from build123d import *

# Parameters (mm, degrees)
F0_R     = 3.175
F1_DEPTH = 12.7
F2_DEPTH = 19.05
F3_R     = 5.08


with BuildPart() as f1:
    # F0 (on Top) → F1 (new body)
    with BuildSketch(Plane.XY):
        with BuildLine():
            Line((21.2967025781, 50.8), (-38.3932974219, 50.8))
            Line((-38.3932974219, 50.8), (-38.3932974219, -6.35))
            Line((-38.3932974219, -6.35), (21.2967025781, -6.35))
            Line((21.2967025781, -6.35), (21.2967025781, -3.175))
            ThreePointArc((21.2967025781, -3.175), (19.0516385478, -2.2450640303), (18.1217025781, 0))
            ThreePointArc((18.1217025781, 0), (21.2967025781, 3.175), (24.4717025781, 0))
            Line((24.4717025781, 0), (31.4567025781, 0))
            Line((31.4567025781, 0), (31.4567025781, 44.45))
            Line((31.4567025781, 44.45), (24.4717025781, 44.45))
            ThreePointArc((24.4717025781, 44.45), (21.2967025781, 41.275), (18.1217025781, 44.45))
            ThreePointArc((18.1217025781, 44.45), (19.0516385478, 46.6950640303), (21.2967025781, 47.625))
            Line((21.2967025781, 47.625), (21.2967025781, 50.8))
        make_face()
        Circle(F0_R, mode=Mode.SUBTRACT)
        with BuildLine():
            ThreePointArc((7.473351289, 0), (10.648351289, 3.175), (13.823351289, 0))
            ThreePointArc((13.823351289, 0), (10.648351289, -3.175), (7.473351289, 0))
        make_face(mode=Mode.SUBTRACT)
        with Locations((0, 44.45)):
            Circle(F0_R, mode=Mode.SUBTRACT)
        with BuildLine():
            ThreePointArc((7.473351289, 44.45), (10.648351289, 47.625), (13.823351289, 44.45))
            ThreePointArc((13.823351289, 44.45), (10.648351289, 41.275), (7.473351289, 44.45))
        make_face(mode=Mode.SUBTRACT)
        with BuildLine():
            Line((31.4567025781, 50.8), (21.2967025781, 50.8))
            Line((21.2967025781, 50.8), (21.2967025781, 47.625))
            ThreePointArc((21.2967025781, 47.625), (23.5417666083, 46.6950640303), (24.4717025781, 44.45))
            Line((24.4717025781, 44.45), (31.4567025781, 44.45))
            Line((31.4567025781, 44.45), (31.4567025781, 50.8))
        make_face()
        with BuildLine():
            Line((21.2967025781, -3.175), (21.2967025781, -6.35))
            Line((21.2967025781, -6.35), (31.4567025781, -6.35))
            Line((31.4567025781, -6.35), (31.4567025781, 0))
            Line((31.4567025781, 0), (24.4717025781, 0))
            ThreePointArc((24.4717025781, 0), (23.5417666083, -2.2450640303), (21.2967025781, -3.175))
        make_face()
    extrude(amount=-F1_DEPTH)

    # F0 (on Top) → F2 (join)
    with BuildSketch(Plane.XY):
        Circle(F0_R)
        with BuildLine():
            ThreePointArc((7.473351289, 0), (10.648351289, -3.175), (13.823351289, 0))
            Line((13.823351289, 0), (7.473351289, 0))
        make_face()
        with BuildLine():
            Line((7.473351289, 0), (13.823351289, 0))
            ThreePointArc((13.823351289, 0), (10.648351289, 3.175), (7.473351289, 0))
        make_face()
        with BuildLine():
            ThreePointArc((24.4717025781, 0), (21.2967025781, 3.175), (18.1217025781, 0))
            Line((18.1217025781, 0), (21.2967025781, 0))
            Line((21.2967025781, 0), (24.4717025781, 0))
        make_face()
        with BuildLine():
            ThreePointArc((18.1217025781, 0), (19.0516385478, -2.2450640303), (21.2967025781, -3.175))
            Line((21.2967025781, -3.175), (21.2967025781, 0))
            Line((21.2967025781, 0), (18.1217025781, 0))
        make_face()
        with BuildLine():
            Line((21.2967025781, 0), (21.2967025781, -3.175))
            ThreePointArc((21.2967025781, -3.175), (23.5417666083, -2.2450640303), (24.4717025781, 0))
            Line((24.4717025781, 0), (21.2967025781, 0))
        make_face()
        with Locations((0, 44.45)):
            Circle(F0_R)
        with BuildLine():
            ThreePointArc((7.473351289, 44.45), (10.648351289, 41.275), (13.823351289, 44.45))
            Line((13.823351289, 44.45), (7.473351289, 44.45))
        make_face()
        with BuildLine():
            Line((7.473351289, 44.45), (13.823351289, 44.45))
            ThreePointArc((13.823351289, 44.45), (10.648351289, 47.625), (7.473351289, 44.45))
        make_face()
        with BuildLine():
            ThreePointArc((24.4717025781, 44.45), (23.5417666083, 46.6950640303), (21.2967025781, 47.625))
            Line((21.2967025781, 47.625), (21.2967025781, 44.45))
            Line((21.2967025781, 44.45), (24.4717025781, 44.45))
        make_face()
        with BuildLine():
            Line((21.2967025781, 44.45), (21.2967025781, 47.625))
            ThreePointArc((21.2967025781, 47.625), (19.0516385478, 46.6950640303), (18.1217025781, 44.45))
            Line((18.1217025781, 44.45), (21.2967025781, 44.45))
        make_face()
        with BuildLine():
            ThreePointArc((18.1217025781, 44.45), (21.2967025781, 41.275), (24.4717025781, 44.45))
            Line((24.4717025781, 44.45), (21.2967025781, 44.45))
            Line((21.2967025781, 44.45), (18.1217025781, 44.45))
        make_face()
    extrude(amount=-F2_DEPTH)

    # F3
    f3_edges = [f1.edges().sort_by_distance(p)[0] for p in [
        (-38.393297, 22.225, 0),
        (-3.468297, -6.35, 0),
        (31.456703, 22.225, 0),
        (-3.468297, 50.8, 0),
    ]]
    fillet(f3_edges, radius=F3_R)


solid = f1.part
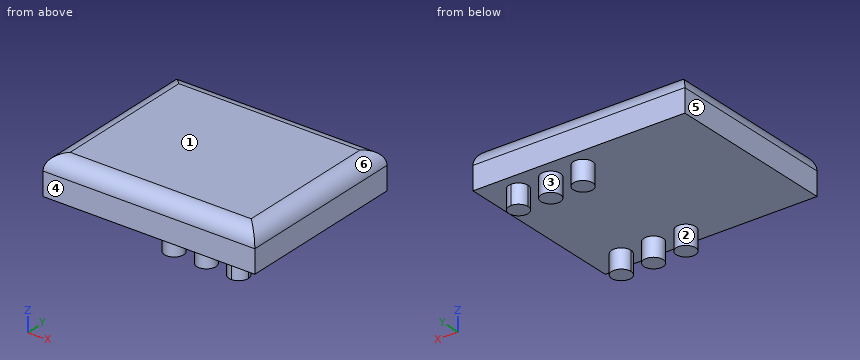
Could you check a few things on this model? Use its own coordinates, in mm. Face numbers are marked on the shaded views. A direction names the side the tool comes from. Give positions to 0.01 mm unless a question says otherwise; leave off trailing zeros. Order: outer loops, then holes, each group sorted by start corner. A loop starts at its lowest first (then second) coordinate and runs counter-clockwise, first axis right, second up. Notation, with made-up numbers: (3, 45.5) - (57, 45.5) arc R21 cw to (57, 83.5) - close; hole circle Ø2 at (-18, 37). An arc over 180 degrees is marked (long way). One line per item, written item: value. Start each with the question number.
1. Imagine slicing it at B-B on x = 0. List the corners of the cut face in (y, z) for me (3 decimals), plus the area to 3 significant figures.
2. For the marked faces 1 and 2, which set-ups out of +Z, -Z, +X, -X, +Y, -Y let a thin tool reach every point of the face, with its end or its side?
3. Imagine slicing it at A-A on z = -17.5. List the corners of the cut face in (x, y) for me (3 decimals).
4. For P1, Ø1, axis at x = -16, z = -4, coming from the -Y side; P2, Ø4, axis at x = 19.5, y = 9, coming from the -Z side, each with a flat end and sliding along its axis, tell me the tip position at first contact or that it passes through.
5. If I drill on probe 1 along X at (y, z) = (45.5, -12.75); probe 2 along X at (y, z) = (2, -17.5); probe 3 along Z at (x, y) = (2, 35), over which ranges is the centre line in solid material (lowest first)?
6. Imagine slicing it at D-D on x = 23.5. List the corners of the cut face in (y, z) for me, plus the area to 3 significant figures.
7. Thinking about a two-plate mould opening in X: for the marked faces 3, 4, 5 and 6, which applies, +X half, -X half, draft (parallel to the pull), parting line (faces both ways), or undercut?
8. Imagine slicing it at C-C on y = 8. List the corners of the cut face in (x, z) for me, plus the area to 3 significant figures.
Values:
1. outline: (-6.35, -12.7) - (-3.175, -12.7) - (-3.175, -19.05) - (3.175, -19.05) - (3.175, -12.7) - (41.275, -12.7) - (41.275, -19.05) - (47.625, -19.05) - (47.625, -12.7) - (50.8, -12.7) - (50.8, -5.08) arc R5.08 ccw to (45.72, 0) - (-1.27, 0) arc R5.08 ccw to (-6.35, -5.08) - close
1. area: 795 mm²
2. face 1: +Z, +X, -X, +Y, -Y
2. face 2: -Z
3. outline: circle Ø6.35 at (0, 0); circle Ø6.35 at (0, 44.45); circle Ø6.35 at (10.648, 0); circle Ø6.35 at (10.648, 44.45); circle Ø6.35 at (21.297, 0); circle Ø6.35 at (21.297, 44.45)
4. P1: y = -6.32
4. P2: z = -12.7
5. probe 1: -3 to 3, 7.65 to 13.64, 18.3 to 24.29
5. probe 2: -2.47 to 2.47, 8.18 to 13.11, 18.83 to 23.76
5. probe 3: -12.7 to 0
6. outline: (-6.35, -12.7) - (-2.29, -12.7) - (-2.29, -19.05) - (2.29, -19.05) - (2.29, -12.7) - (42.16, -12.7) - (42.16, -19.05) - (46.74, -19.05) - (46.74, -12.7) - (50.8, -12.7) - (50.8, -5.08) arc R5.08 ccw to (45.72, 0) - (-1.27, 0) arc R5.08 ccw to (-6.35, -5.08) - close
6. area: 773 mm²
7. face 3: undercut
7. face 4: draft
7. face 5: -X half
7. face 6: +X half
8. outline: (-38.39, -12.7) - (31.46, -12.7) - (31.46, -5.08) arc R5.08 ccw to (26.38, 0) - (-33.31, 0) arc R5.08 ccw to (-38.39, -5.08) - close
8. area: 876 mm²
